Job drawing, mm, ordinate dimensions from the low corner. One solid piece. A direction names the side the tool comes from. Round coordinates to 2 decimals unless told otherwise and drop trailing zeros. Order: outer loops, then holes, each group sorted by start corner. A loop starts at its lowest first (then second) coordinate and runs counter-clockwise, first axis right, second up. Notation, with made-up numbers: (68, 39.5) -> (88, 39.5) arc R20 ccw to (88, 77.5) -> close; hole circle Ø11 at (-39, 0.5). An arc over 180 degrees is marked (long way). Return JSON: item names as keys, results as strings. Group by question number.
Q1. Which spindle directions (+Z, -Z, +X, -X, +Y, -Y) get a long thin tool onto all of the face, cutting with end or side? Do the marked faces 5, 6, 7, 8 and 9. Say none if no direction does.
Q2. Probe line 1 along X through (y, z) = (59, 34); line 2 along X through (y, z) = (41, 41.5); line 3 along Z through (x, y) = (131, 83.5). List the from-to ranges inside material, lowest first.
Q3. Cut at C-C (z = 11). Write the cut outline in (x, y), then the cut area to 3 significant figures.
Q4. Mould opens along X. For the marked faces 1, 2, 3 and 4 say: +X half, -X half, draft (parallel to the pull), parting line (faces both ways), or undercut.
Q5. Cut at B-B (x = 133). Write the cut outline in (y, z), then the cut area to 3 significant figures.
Q6. Flat gauge pins, fed straight in: pin 1 (1.5 mm diameter, centred on x = 87, y = 35, fed in from +Z); pin 2 (7.5 mm diameter, centred on x = 19, y = 41.5, fed in from +Z). Where does each tip first touch, or does it go through?
Q7. Cut at A-A (y = 43.5). Write the cut outline in (x, z), then the cut area to 3 significant figures.
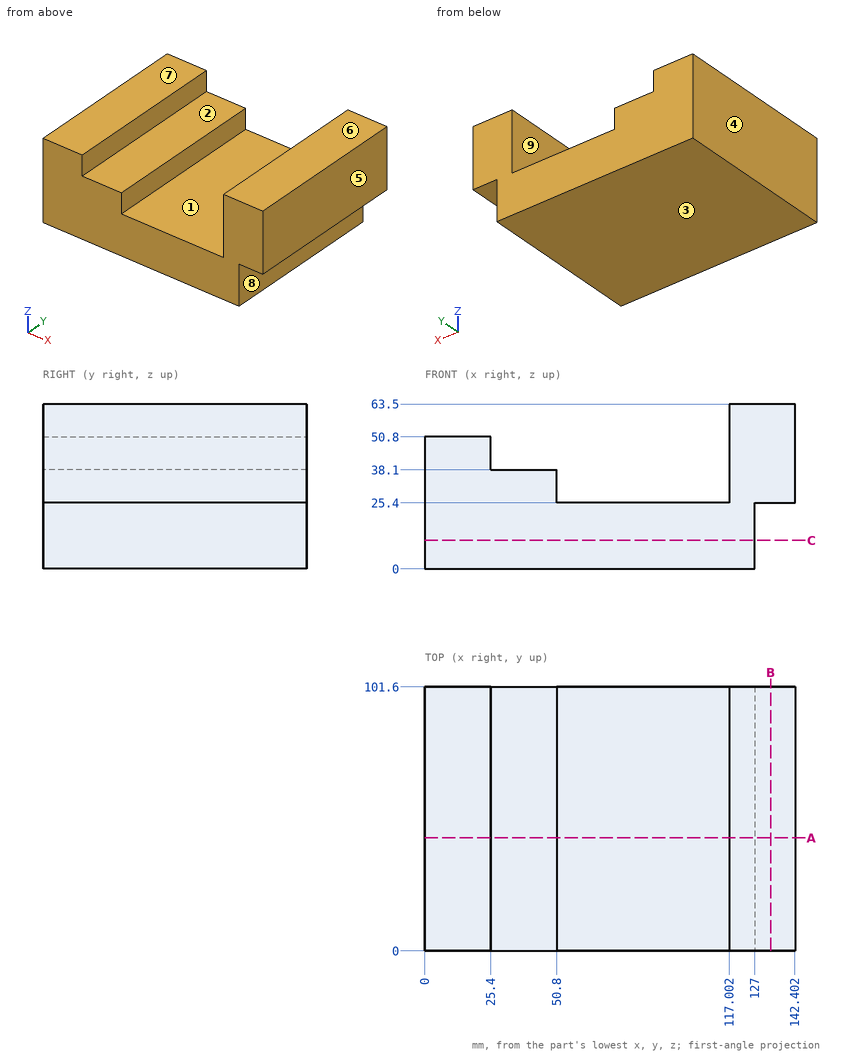
Solution:
{
 "1": {"face 5": "+Z, -Z, +X, +Y, -Y", "face 6": "+Z, +X, -X, +Y, -Y", "face 7": "+Z, -X, +Y, -Y", "face 8": "-Z, +X, +Y, -Y", "face 9": "+Z, +Y, -Y"},
 "2": {"line 1": "x = 0 to 50.8, 117 to 142.4", "line 2": "x = 0 to 25.4, 117 to 142.4", "line 3": "z = 25.4 to 63.5"},
 "3": {"outline": "(0, 0) -> (127, 0) -> (127, 101.6) -> (0, 101.6) -> close", "area": "12,900 mm²"},
 "4": {"face 1": "undercut", "face 2": "undercut", "face 3": "draft", "face 4": "-X half"},
 "5": {"outline": "(0, 25.4) -> (101.6, 25.4) -> (101.6, 63.5) -> (0, 63.5) -> close", "area": "3,870 mm²"},
 "6": {"pin 1": "stops at z = 25.4", "pin 2": "stops at z = 50.8"},
 "7": {"outline": "(0, 0) -> (127, 0) -> (127, 25.4) -> (142.4, 25.4) -> (142.4, 63.5) -> (117, 63.5) -> (117, 25.4) -> (50.8, 25.4) -> (50.8, 38.1) -> (25.4, 38.1) -> (25.4, 50.8) -> (0, 50.8) -> close", "area": "5,160 mm²"}
}
